Verification items for the finished model (mm, model axes). A direction names the side the tool comes from. Give positions to 0.01 mm unless a question says otherwise; leave off trailing zeros. Order: outer loops, then holes, each group sorted by start corner. A loop starts at its lowest first (then second) coordinate and runs counter-clockwise, first axis right, second up.
(1) Sectioned sample at C-C on x = 40. Record the cut outline in (y, z), plus the area to 3 significant figures.
(2) Sectioned sample at D-D on x = -17.5. Record the cut outline in (y, z), plus the area to 3 significant figures.
(3) Scan lines: L1, parallel to Y at x = -39, z = 0.15; L2, parallel to X at y = 0.5, z = 2.65; L3, parallel to Z at x = -1, y = -0.85. Record each from-to range of solid material in increasing order.
(4) Sectioned sample at A-A on z = 0. Record the cut outline in (x, y).
(5) Gauge pin test, flat ends, axial feed: pin 1 (2 mm diameter, centred on x = 8, z = -1.5, fed in from -Y); pin 2 (1 mm diameter, centred on x = -30, y = 1.5, fed in from -Z). Record the tip position at first contact, or that the pin passes through.
(6) Access from +Z, -Z, +X, -X, +Y, -Y to the whole of each face (thin tool, end or side, straight path). Record for faces 1 (the face through (41, -2, 0)), 2 (the face through (-35, -2, -1)), 3 (the face through (-46.75, 0, 0)).
```python
from build123d import *

# Parameters (mm, degrees)
BOSS_EXTRUDE1_DEPTH      = 35
BOSS_EXTRUDE1_DEPTH_BACK = 35
SKETCH1_R                = 3
BOSS_EXTRUDE2_DEPTH      = 46.75
BOSS_EXTRUDE2_DEPTH_BACK = 46.75
SKETCH3_R                = 2


with BuildPart() as part:
    # Sketch1 → Boss-Extrude1 (new, two sides: drawn at the far end of the back side and taken through both)
    with BuildSketch(Plane(origin=(0, 0, 0), x_dir=(0, 0, -1), z_dir=(1, 0, 0)).offset(-BOSS_EXTRUDE1_DEPTH_BACK)):
        Circle(SKETCH1_R)
    extrude(amount=BOSS_EXTRUDE1_DEPTH + BOSS_EXTRUDE1_DEPTH_BACK)

    # Sketch3 → Boss-Extrude2 (add, two sides: drawn at the far end of the back side and taken through both)
    with BuildSketch(Plane(origin=(0, 0, 0), x_dir=(0, 0, -1), z_dir=(1, 0, 0)).offset(-BOSS_EXTRUDE2_DEPTH_BACK)):
        Circle(SKETCH3_R)
    extrude(amount=BOSS_EXTRUDE2_DEPTH + BOSS_EXTRUDE2_DEPTH_BACK)


solid = part.part
```
Ans:
1. outline: circle Ø4 at (0, 0)
1. area: 12.6 mm2
2. outline: circle Ø6 at (0, 0)
2. area: 28.3 mm2
3. L1: y = -1.99 to 1.99
3. L2: x = -35 to 35
3. L3: z = -2.88 to 2.88
4. outline: (-46.75, -2) - (-35, -2) - (-35, -3) - (35, -3) - (35, -2) - (46.75, -2) - (46.75, 2) - (35, 2) - (35, 3) - (-35, 3) - (-35, 2) - (-46.75, 2) - close
5. pin 1: stops at y = -2.96
5. pin 2: stops at z = -2.83
6. face 1: +X
6. face 2: -X
6. face 3: +Z, -Z, -X, +Y, -Y
